The listing builds one solid part. Answer for the finished solid, in the listing's coordinates (mm). A direction names the side the tool comes from. Coordinates: 2 decimals unless noted, no trailing zeros. Loops run counter-clockwise (first coordinate to the right, second up) from the corner with the lowest first, then second, coordinate; pieces in that order, holes last. Notation, with made-up numbers: (-7.5, -19.75) -> (29.5, -19.75) arc R29 ccw to (29.5, 14.25) -> close; hole circle Ø7 at (76, -31.75). An arc over 180 degrees is marked (long way). Answer in a Markdown table with one row per item.
```python
from build123d import *

# Parameters (mm, degrees)
CROQUIS1_R              = 2.5
SALIENTE_EXTRUIR1_DEPTH = 480
CUT_EXTRUDE1_DEPTH      = 25
CUT_EXTRUDE1_DEPTH_BACK = 24
SKETCH2_W               = 600
SKETCH2_H               = 26.97008712
CUT_EXTRUDE4_DEPTH      = 21
CUT_EXTRUDE4_DEPTH_BACK = 41
SKETCH4_W               = 140
SKETCH4_H               = 71.605139047


with BuildPart() as part:
    # Croquis1 → Saliente-Extruir1 (new body)
    with BuildSketch(Plane.XY):
        with BuildLine():
            Line((-4.6, 10), (-3.1, 8.5))
            Line((-3.1, 8.5), (-3.1, 8.2))
            Line((-3.1, 8.2), (-5.5, 8.2))
            Line((-5.5, 8.2), (-5.5, 6.560660172))
            Line((-5.5, 6.560660172), (-2.84, 3.900660172))
            Line((-2.84, 3.900660172), (0, 3.900660172))
            Line((0, 3.900660172), (2.84, 3.900660172))
            Line((2.84, 3.900660172), (5.5, 6.560660172))
            Line((5.5, 6.560660172), (5.5, 8.2))
            Line((5.5, 8.2), (3.1, 8.2))
            Line((3.1, 8.2), (3.1, 8.5))
            Line((3.1, 8.5), (4.6, 10))
            Line((4.6, 10), (9.25, 10))
            ThreePointArc((9.25, 10), (9.780330086, 9.780330086), (10, 9.25))
            Line((10, 9.25), (10, 4.6))
            Line((10, 4.6), (8.5, 3.1))
            Line((8.5, 3.1), (8.2, 3.1))
            Line((8.2, 3.1), (8.2, 5.5))
            Line((8.2, 5.5), (6.560660172, 5.5))
            Line((6.560660172, 5.5), (3.900660172, 2.84))
            Line((3.900660172, 2.84), (3.900660172, 0))
            Line((3.900660172, 0), (3.900660172, -2.84))
            Line((3.900660172, -2.84), (6.560660172, -5.5))
            Line((6.560660172, -5.5), (8.2, -5.5))
            Line((8.2, -5.5), (8.2, -3.1))
            Line((8.2, -3.1), (8.5, -3.1))
            Line((8.5, -3.1), (10, -4.6))
            Line((10, -4.6), (10, -9.25))
            ThreePointArc((10, -9.25), (9.780330086, -9.780330086), (9.25, -10))
            Line((9.25, -10), (4.6, -10))
            Line((4.6, -10), (3.1, -8.5))
            Line((3.1, -8.5), (3.1, -8.2))
            Line((3.1, -8.2), (5.5, -8.2))
            Line((5.5, -8.2), (5.5, -6.560660172))
            Line((5.5, -6.560660172), (2.84, -3.900660172))
            Line((2.84, -3.900660172), (0, -3.900660172))
            Line((0, -3.900660172), (-2.84, -3.900660172))
            Line((-2.84, -3.900660172), (-5.5, -6.560660172))
            Line((-5.5, -6.560660172), (-5.5, -8.2))
            Line((-5.5, -8.2), (-3.1, -8.2))
            Line((-3.1, -8.2), (-3.1, -8.5))
            Line((-3.1, -8.5), (-4.6, -10))
            Line((-4.6, -10), (-9.25, -10))
            ThreePointArc((-9.25, -10), (-9.780330086, -9.780330086), (-10, -9.25))
            Line((-10, -9.25), (-10, -4.6))
            Line((-10, -4.6), (-8.5, -3.1))
            Line((-8.5, -3.1), (-8.2, -3.1))
            Line((-8.2, -3.1), (-8.2, -5.5))
            Line((-8.2, -5.5), (-6.560660172, -5.5))
            Line((-6.560660172, -5.5), (-3.900660172, -2.84))
            Line((-3.900660172, -2.84), (-3.900660172, 0))
            Line((-3.900660172, 0), (-3.900660172, 2.84))
            Line((-3.900660172, 2.84), (-6.560660172, 5.5))
            Line((-6.560660172, 5.5), (-8.2, 5.5))
            Line((-8.2, 5.5), (-8.2, 3.1))
            Line((-8.2, 3.1), (-8.5, 3.1))
            Line((-8.5, 3.1), (-10, 4.6))
            Line((-10, 4.6), (-10, 9.25))
            ThreePointArc((-10, 9.25), (-9.780330086, 9.780330086), (-9.25, 10))
            Line((-9.25, 10), (-4.6, 10))
        make_face()
        Circle(CROQUIS1_R, mode=Mode.SUBTRACT)
    extrude(amount=SALIENTE_EXTRUIR1_DEPTH)

    # Sketch2 → Cut-Extrude1 (cut, two sides: drawn at the far end of the back side and taken through both)
    with BuildSketch(Plane(origin=(0, 0, 0), x_dir=(0, 0, -1), z_dir=(1, 0, 0)).offset(-CUT_EXTRUDE1_DEPTH_BACK)):
        Rectangle(SKETCH2_W, SKETCH2_H)
    extrude(amount=CUT_EXTRUDE1_DEPTH + CUT_EXTRUDE1_DEPTH_BACK, mode=Mode.SUBTRACT)

    # Sketch4 → Cut-Extrude4 (cut, two sides: drawn at the far end of the back side and taken through both)
    with BuildSketch(Plane(origin=(0, 0, 0), x_dir=(0, 0, -1), z_dir=(1, 0, 0)).offset(-CUT_EXTRUDE4_DEPTH_BACK)):
        with Locations((-365, -0.774109611)):
            Rectangle(SKETCH4_W, SKETCH4_H)
    extrude(amount=CUT_EXTRUDE4_DEPTH + CUT_EXTRUDE4_DEPTH_BACK, mode=Mode.SUBTRACT)


solid = part.part
```
Item 1: Flat-ended cylindrical pins translate along their axes: pin 1 Ø2 at (y, z) = (-3.5, 474) entering from -X; pin 2 Ø2 at (x, y) = (3, -6.5) entering from +Z; pin 3 Ø1.7 at (x, z) = (1, 447.5) entering from +Y. Find the tip coordinate at first contact, or state that the pin passes through.
Findings below:
| item | result |
|---|---|
| pin 1 | stops at x = -9.9 |
| pin 2 | passes through |
| pin 3 | stops at y = 3.9 |
Item 2: Determine the mould class of faces 1 (the face through (-9.2, 3.8, 457.2)), 2 (the face through (-5.25, -4.19, 457.18)), 3 (the face through (7, -10, 457)), 4 (the face through (5.21, -4.15, 457.18)) for opening direction X: +X half, -X half, draft (parallel to the pull), parting line (faces both ways), or undercut.
Findings below:
| item | result |
|---|---|
| face 1 | -X half |
| face 2 | undercut |
| face 3 | draft |
| face 4 | undercut |
Item 3: A cutting plane is placed at A-A, the plane y = 0. Determine the outline of the cut face in (x, z).
Findings below:
| item | result |
|---|---|
| outline | (-3.9, 435) -> (-2.5, 435) -> (-2.5, 480) -> (-3.9, 480) -> close; (2.5, 435) -> (3.9, 435) -> (3.9, 480) -> (2.5, 480) -> close |
Item 4: Find the intervals of material crossed by probe 1 along X at (y, z) = (7, 441.5); probe 2 along X at (y, z) = (0, 444.5), in increasing order.
Findings below:
| item | result |
|---|---|
| probe 1 | x = -10 to -5.5, 5.5 to 10 |
| probe 2 | x = -3.9 to -2.5, 2.5 to 3.9 |
Item 5: A tool of negligible diameter and unlimited length cuts with its end or side. For faces 5 (the face through (-3.8, -9.2, 457.2)), 6 (the face through (-10, -7, 457)), 7 (the face through (5.25, 4.19, 457.18)), 8 (the face through (0, 3.901, 457)), 9 (the face through (-7, 10, 457)), from which of +Z, -Z, +X, -X, +Y, -Y can it reach the whole face along a straight path? Write none if from no direction.
Findings below:
| item | result |
|---|---|
| face 5 | +Z, -Z, -Y |
| face 6 | +Z, -Z, -X, +Y, -Y |
| face 7 | +Z, -Z |
| face 8 | +Z, -Z, +Y |
| face 9 | +Z, -Z, +X, -X, +Y |
